CAD build for the part. Positions are in the model's coordinates, mm. Face numbers are marked on the shaded views. Coordinates: 2 decimals unless noted, no trailing zeros. Order: outer loops, then holes, each group sorted by start corner. A loop starts at its lowest first (then second) coordinate and runs counter-clockwise, first axis right, second up. Notation, with made-up numbers: (41.25, 41.5) - (83.25, 41.5) arc R21 cw to (83.25, 46.5) - close; hole circle Ø4 at (42.5, 29.25). An arc over 180 degrees is marked (long way). Write each question's results on one line, items separated by ' | '. Start each with the question number.
Q1. Band-saw the part on A-A, the plane z = 17.5. Write the cut outline in (x, y), then the cut area to 3 significant figures.
Q2. Wall check: probe 1 along Z at (x, y) = (1.75, 17.5); probe 2 along Y at (x, z) = (0.5, 19.5); probe 3 along Y at (x, z) = (-1.5, 25.5). Give the ranges that are in metal, low to high.
Q3. Pull direction Y, two halves, no side cores. Call the marked faces 1, 2 and 3: released by +Y, released by -Y, zero draft, split by the parting line, or undercut.
Q4. Band-saw the part on C-C, the plane x = 1. Write the cut outline in (y, z).
```python
from build123d import *

# Parameters (mm, degrees)
SKETCH_W    = 35
SKETCH_H    = 35
SKETCH_R    = 12.5
PAD_DEPTH   = 3.25
SKETCH001_R = 1.5
HOLE_DEPTH  = 25


with BuildPart() as part:
    # Sketch → Pad (new body, symmetric)
    with BuildSketch(Plane.YZ):
        with Locations((17.5, 17.5)):
            Rectangle(SKETCH_W, SKETCH_H)
        with Locations((17.5, 17.5)):
            Circle(SKETCH_R, mode=Mode.SUBTRACT)
    extrude(amount=PAD_DEPTH, both=True)

    # Sketch001 (on Face6 of Pad) → Hole (cut)
    with BuildSketch(Plane(origin=(-3.25, 0, 0), x_dir=(0, 1, 0), z_dir=(-1, 0, 0))):
        with Locations((30, -30)):
            Circle(SKETCH001_R)
        with Locations((5, -5)):
            Circle(SKETCH001_R)
        with Locations((30, -5)):
            Circle(SKETCH001_R)
        with Locations((5, -30)):
            Circle(SKETCH001_R)
    extrude(amount=-HOLE_DEPTH, mode=Mode.SUBTRACT)


solid = part.part
```
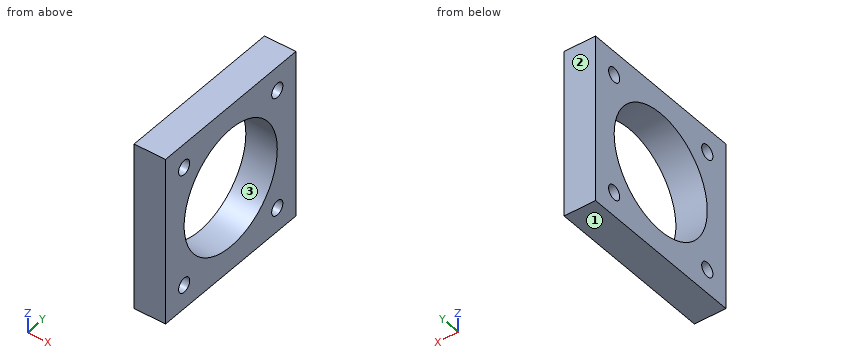
Results below:
1) outline: (-3.25, 0) - (3.25, 0) - (3.25, 5) - (-3.25, 5) - close; (-3.25, 30) - (3.25, 30) - (3.25, 35) - (-3.25, 35) - close | area: 65.0 mm²
2) probe 1: z = 0 to 5, 30 to 35 | probe 2: y = 0 to 5.16, 29.84 to 35 | probe 3: y = 0 to 7.9, 27.1 to 35
3) face 1: zero draft | face 2: released by +Y | face 3: undercut
4) outline: (0, 0) - (35, 0) - (35, 35) - (0, 35) - close; hole circle Ø3 at (5, 5); hole circle Ø3 at (5, 30); hole circle Ø25 at (17.5, 17.5); hole circle Ø3 at (30, 5); hole circle Ø3 at (30, 30)
